The listing builds one solid part. Answer for the finished solid, in the listing's coordinates (mm). Face numbers are marked on the shaded views. A direction names the side the tool comes from. Coordinates: 2 decimals unless noted, no trailing zeros. Write each loop counter-clockwise with the first axis right and the second up, starting at its lowest first coordinate (ties: lowest second). Pieces come first, ordered by that corner, then holes. Notation, with made-up numbers: M -26.75,-34.75 L 23.25,-34.75 A20 ccw 23.25,-10.75 Z; hole C -0.75,39.25 d2. An arc over 180 degrees is marked long. Put each result on its own line as item: value. Start each with the question number.
```python
from build123d import *

# Parameters (mm, degrees)
CUT_EXTRUDE1_DEPTH = 0.75
SKETCH3_R          = 5.4
CUT_EXTRUDE2_DEPTH = 1
SKETCH4_R          = 4.85
CUT_EXTRUDE3_DEPTH = 1
SKETCH5_R          = 6.75
CUT_EXTRUDE4_DEPTH = 2.2


with BuildPart() as part:
    # Sketch1 → Revolve1 (revolve)
    with BuildSketch(Plane(origin=(0, 0, 0), x_dir=(0, 0, -1), z_dir=(1, 0, 0))):
        Polygon((0, 0), (0, 7.5), (16.4, 8.8), (30.9, 9), (45.4, 9), (45.4, 7.5), (57.76, 7.5), (57.76, 6.125), (58.51, 6.125), (58.51, 0), align=None)
    revolve(axis=Axis((0, 0, -58.51), (0, 0, 1)))

    # Sketch2 → Cut-Extrude1 (cut)
    with BuildSketch(Plane(origin=(0, 0, -58.51), x_dir=(-1, 0, 0), z_dir=(0, 0, -1))):
        with BuildLine():
            Line((-3.836013556, 4.775), (3.836013556, 4.775))
            ThreePointArc((3.836013556, 4.775), (0, 6.125), (-3.836013556, 4.775))
        make_face()
    extrude(amount=-CUT_EXTRUDE1_DEPTH, mode=Mode.SUBTRACT)

    # Sketch3 → Cut-Extrude2 (cut)
    with BuildSketch(Plane.XY):
        Circle(SKETCH3_R)
    extrude(amount=-CUT_EXTRUDE2_DEPTH, mode=Mode.SUBTRACT)

    # Sketch4 → Cut-Extrude3 (cut)
    with BuildSketch(Plane.XY.offset(-1)):
        Circle(SKETCH4_R)
    extrude(amount=-CUT_EXTRUDE3_DEPTH, mode=Mode.SUBTRACT)

    # Sketch5 → Cut-Extrude4 (cut)
    with BuildSketch(Plane.XY.offset(-2)):
        Circle(SKETCH5_R)
    extrude(amount=-CUT_EXTRUDE4_DEPTH, mode=Mode.SUBTRACT)


solid = part.part
```
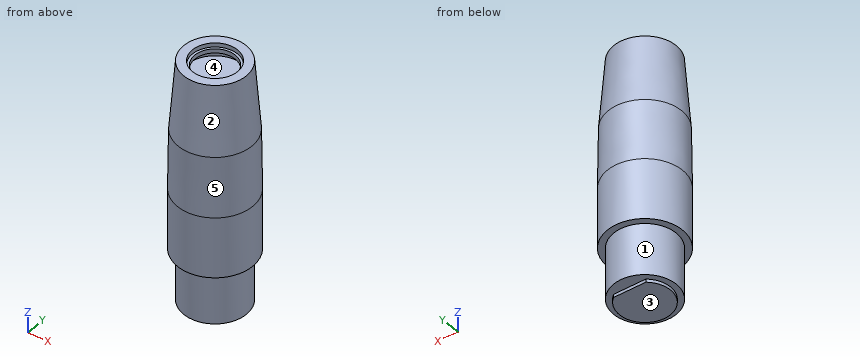
1) Determine the mould class of the marked faces 3, 4 and 5 for opening direction Z: +Z half, -Z half, draft (parallel to the pull), parting line (faces both ways), or undercut.
2) For the marked faces 1 and 2, determine the directions among +Z, -Z, +X, -X, +Y, -Y from which every point of the face is accessible in a straight line to the end or side of a thin tool.
3) Given pin 1 Ø4 at (x, y) = (7, 5.5) entering from -Z; pin 2 Ø10 at (x, z) = (6.5, -27) entering from -Y; pin 3 Ø2 at (x, z) = (1.5, -24) entering from +Y, each flat-ended and moving along its own axis, determine where each tip first touches the part or whether it passes through.
4) A cutting plane is placed at B-B on z = -17. Write down the section's boundary in (x, y).
5) Straight lines are drawn through the part: probe 1 along Z at (x, y) = (-2.5, -4.5); probe 2 along Y at (x, z) = (0, -1.2); probe 3 along Z at (x, y) = (3, -3.75). For each, find the intervals that lie inside material, in ascending order.
6) A cutting plane is placed at A-A on z = -40. Write down the section's boundary in (x, y).
Answers follow:
1. face 3: -Z half
1. face 4: undercut
1. face 5: +Z half
2. face 1: -Z
2. face 2: +Z
3. pin 1: stops at z = -57.76
3. pin 2: stops at y = -8.82
3. pin 3: stops at y = 8.89
4. outline: C 0,0 d17.62
5. probe 1: z = -58.51 to -4.2, -2 to -1
5. probe 2: y = -7.6 to -4.85, 4.85 to 7.6
5. probe 3: z = -58.51 to -4.2
6. outline: C 0,0 d18
